Check sheet for the drawn part. Datum: minimum x, y, z corner. Units: mm. Give positions to 0.01 mm unless a question says otherwise; leave off trailing zeros. Order: outer loops, then holes, each group sorted by start corner. A loop starts at its lowest first (then second) coordinate and runs counter-clockwise, first axis right, second up. Notation, with made-up numbers: M 75.25,19.25 L 133.25,19.25 A21 ccw 133.25,56.25 Z; hole C -34.5,85.25 d9. An arc over 180 degrees is marked long. One line per question, with ' | ' between items. Start each with the question number.
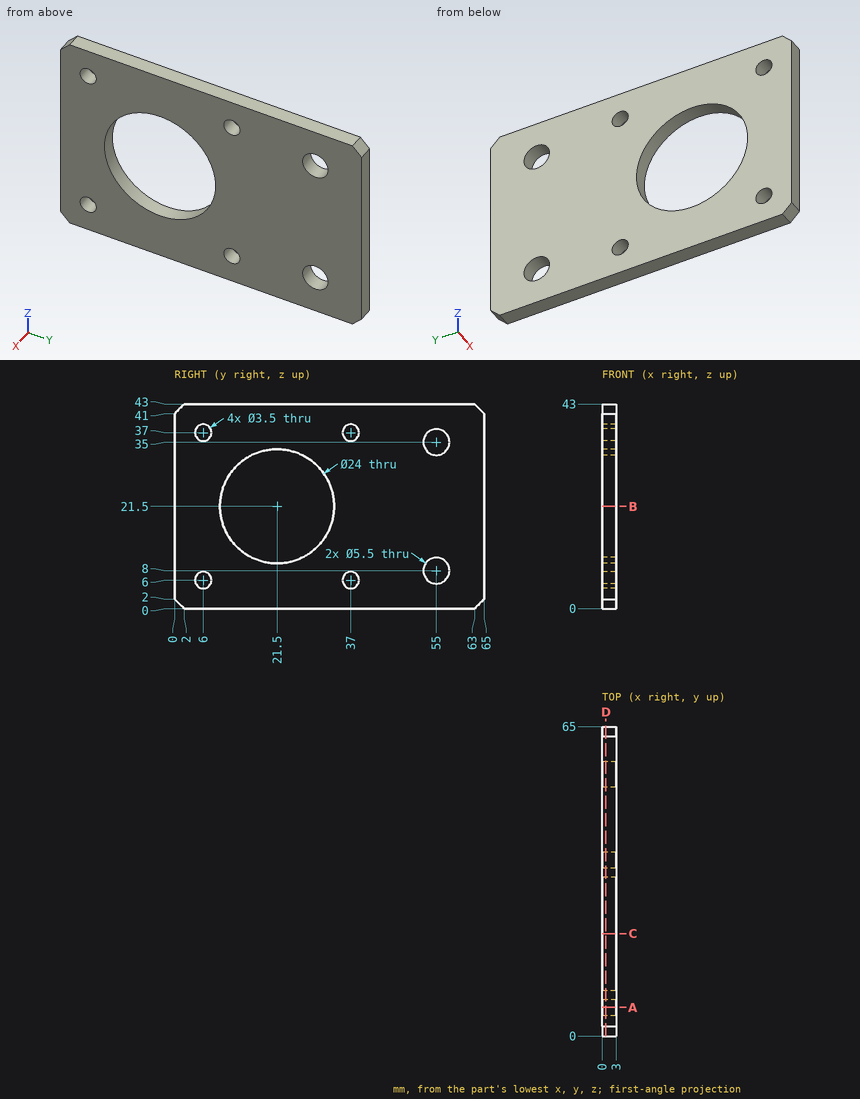
Item 1: Section check C-C, the plane y = 21.5. Record the cut outline in (x, z).
Item 2: Scan lines: probe 1 along Z at (x, y) = (1.7, 37); probe 2 along Z at (x, y) = (2.45, 55); probe 3 along Y at (x, z) = (1.65, 21.5). Record each from-to range of solid material in increasing order. Write a range as [from, to].
Item 3: Section check D-D, the plane x = 0.8. Record the cut outline in (y, z).
Item 4: Section check B-B, the plane z = 21.5. Record the cut outline in (x, y), then the cut area to 3 significant figures.
Item 5: Go/stop test with a flat-tipped pin: P1, Ø6.5, axis at y = 55, z = 35, coming from the -X side. Record where the tip stops, or that it passes through.
Item 6: Section check A-A, the plane y = 6. Record the cut outline in (x, z), then the cut area to 3 significant figures.
Reported:
1) outline: M 0,0 L 3,0 L 3,9.5 L 0,9.5 Z; M 0,33.5 L 3,33.5 L 3,43 L 0,43 Z
2) probe 1: z = [0, 4.25], [7.75, 35.25], [38.75, 43] | probe 2: z = [0, 5.25], [10.75, 32.25], [37.75, 43] | probe 3: y = [0, 9.5], [33.5, 65]
3) outline: M 0,2 L 2,0 L 63,0 L 65,2 L 65,41 L 63,43 L 2,43 L 0,41 Z; hole C 6,6 d3.5; hole C 6,37 d3.5; hole C 21.5,21.5 d24; hole C 37,6 d3.5; hole C 37,37 d3.5; hole C 55,8 d5.5; hole C 55,35 d5.5
4) outline: M 0,0 L 3,0 L 3,9.5 L 0,9.5 Z; M 0,33.5 L 3,33.5 L 3,65 L 0,65 Z | area: 123 mm^2
5) P1: stops at x = 0
6) outline: M 0,0 L 3,0 L 3,4.25 L 0,4.25 Z; M 0,7.75 L 3,7.75 L 3,35.25 L 0,35.25 Z; M 0,38.75 L 3,38.75 L 3,43 L 0,43 Z | area: 108 mm^2
